Verification items for the finished model (mm, model axes). A direction names the side the tool comes from. Round coordinates to 2 decimals unless told otherwise and drop trailing zeros. Order: outer loops, then holes, each group sorted by start corner. A loop starts at its lowest first (then second) coordinate and runs counter-clockwise, first axis right, second up. Notation, with made-up numbers: (48, 42.25) -> (91, 42.25) arc R15 ccw to (91, 71.25) -> close; hole circle Ø6 at (65.5, 64.5). An arc over 180 degrees is marked (long way). Return JSON: item names as keys, results as strings. Group by question number.
Item 1: Sectioned sample at A-A on y = 0. Record the cut outline in (x, z), plus the area to 3 significant figures.
Item 2: Sectioned sample at C-C on z = 24.5. Record the cut outline in (x, y).
Item 3: Scan lines: probe 1 along Y at (x, z) = (-0.5, 41.5); probe 2 along X at (y, z) = (-0.5, 44.5); probe 3 along Y at (x, z) = (-6.5, 41). Record each from-to range of solid material in increasing order. Write a range as from..to.
Item 4: Draft check along Y on faces 4 (the flat face through (-15.809, -33, 30)), 5 (the cylindrical face through (56.246, 17.713, 56.155)), 6 (the flat face through (28, 1, 0)). Enter one of: pulls with the +Y half, pulls with the -Y half, needs draft (parallel to the pull), parting line crosses it, or undercut.
Item 5: Sectioned sample at B-B on x = -11. Record the cut outline in (y, z), plus the area to 3 significant figures.
Item 6: Sectioned sample at D-D on y = 56. Record the cut outline in (x, z), plus the area to 3 significant figures.
Item 7: Depth check by flat-ended pin: pin 1 Ø1.5 at (x, z) = (-6, 45) entering from +Y; pin 2 Ø7 at (y, z) = (-31, 34.5) entering from +X; pin 3 Ø10 at (y, z) = (30.5, 43) entering from -X. Enter the tip coordinate at first touch or a pass-through.
Item 8: Access from +Z, -Z, +X, -X, +Y, -Y to the whole of each face (thin tool, end or side, straight path). Record for faces 1 (the flat face through (15.888, -34, 30)), 2 (the flat face through (-1, 27, 59.4)), 3 (the flat face through (-49, -34, 53)).
```python
from build123d import *

# Parameters (mm, degrees)
F0_R     = 65.258808
F1_DEPTH = 53
F2_R     = 58.968994
F3_DEPTH = 6.4
F5_DEPTH = 73.5


with BuildPart() as f1:
    # F0 (on Top) → F1 (new body)
    with BuildSketch(Plane.XY):
        Circle(F0_R)
    extrude(amount=F1_DEPTH)

    # F2 (on face) → F3 (join)
    with BuildSketch(Plane.XY.offset(53)):
        Circle(F2_R)
    extrude(amount=F3_DEPTH)

    # F4 (on face) → F5 (cut)
    with BuildSketch(Plane.XY.offset(59.4)):
        with BuildLine():
            Line((15.88816, -21.688723), (15.809092, -21.688723))
            ThreePointArc((15.809092, -21.688723), (0, 26.838929), (-15.809092, -21.688723))
            Line((-15.809092, -21.688723), (-15.809092, -45.453947))
            Line((-15.809092, -45.453947), (15.88816, -45.453947))
            Line((15.88816, -45.453947), (15.88816, -21.688723))
        make_face()
    extrude(amount=-F5_DEPTH, mode=Mode.SUBTRACT)


solid = f1.part
```
Recorded:
{
 "1": {"outline": "(-65.26, 0) -> (-26.84, 0) -> (-26.84, 59.4) -> (-58.97, 59.4) -> (-58.97, 53) -> (-65.26, 53) -> close; (26.84, 0) -> (65.26, 0) -> (65.26, 53) -> (58.97, 53) -> (58.97, 59.4) -> (26.84, 59.4) -> close", "area": "4,480 mm²"},
 "2": {"outline": "circle Ø130.52 at (0, 0); hole (-15.81, -45.45) -> (15.89, -45.45) -> (15.89, -21.69) -> (15.81, -21.69) arc R26.84 ccw (long way) to (-15.81, -21.69) -> close"},
 "3": {"probe 1": "-65.26..-45.45, 26.83..65.26", "probe 2": "-65.26..-26.83, 26.83..65.26", "probe 3": "-64.93..-45.45, 26.04..64.93"},
 "4": {"face 4": "undercut", "face 5": "parting line crosses it", "face 6": "needs draft"},
 "5": {"outline": "(-64.33, 0) -> (-45.45, 0) -> (-45.45, 59.4) -> (-57.93, 59.4) -> (-57.93, 53) -> (-64.33, 53) -> close; (24.48, 0) -> (64.33, 0) -> (64.33, 53) -> (57.93, 53) -> (57.93, 59.4) -> (24.48, 59.4) -> close", "area": "3,410 mm²"},
 "6": {"outline": "(-33.51, 0) -> (33.51, 0) -> (33.51, 53) -> (18.48, 53) -> (18.48, 59.4) -> (-18.48, 59.4) -> (-18.48, 53) -> (-33.51, 53) -> close", "area": "3,790 mm²"},
 "7": {"pin 1": "y = 65.05", "pin 2": "x = 59.18", "pin 3": "x = -60.07"},
 "8": {"face 1": "+Z, -Z", "face 2": "+Z, +X, -X, +Y, -Y", "face 3": "+Z"}
}
